Could you check a few things on this drawing? It's one solid part, dimensions in mm from its lowest x, y, z. A direction names the side the tool comes from. Round coordinates to 2 decimals unless told otherwise and drop trailing zeros. Order: outer loops, then holes, each group sorted by start corner. A loop starts at its lowest first (then second) coordinate and runs counter-clockwise, first axis right, second up.
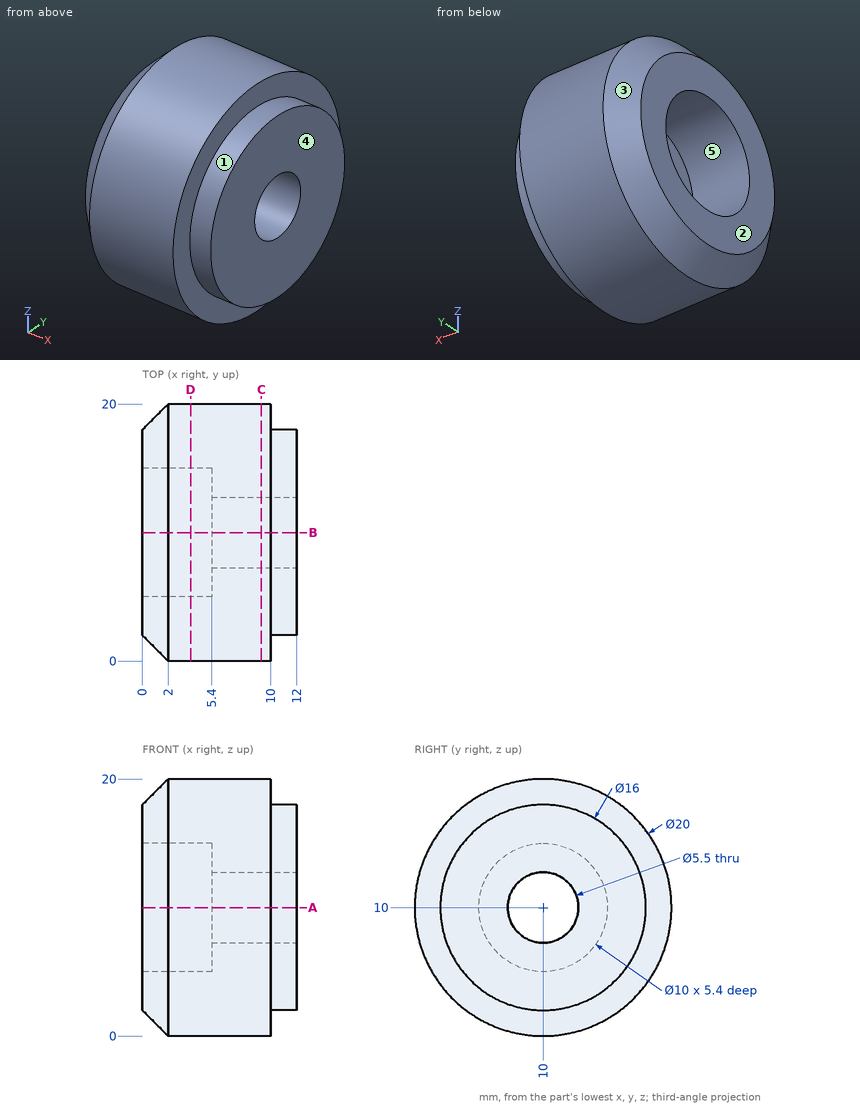
(1) On a 3-axis mill with a long thin cutter (end or side, diameter ignored), from which of +Z, -Z, +X, -X, +Y, -Y can I reach the whole of each face in a straight line? I mean the marked faces 1 and 2. Say none if no direction works.
(2) I'm going to push flat-ended pins straight in: pin 1 Ø3 at (x, y) = (3.5, 17.5) entering from -Z; pin 2 Ø2 at (y, z) = (16, 17) entering from +X; pin 3 Ø3 at (y, z) = (12, 8.5) entering from -X. Where does each tip first touch, or does it pass through?
(3) I want a section at C-C, the plane x = 9.25. List the corners of the cut face in (y, z) for me, plus the area to 3 significant figures.
(4) I want a section at D-D, the plane x = 3.75. List the corners of the cut face in (y, z) for me.
(5) Please list where these lines run through material, in increasing order: probe 1 along Y at (x, z) = (10.5, 10); probe 2 along Y at (x, z) = (7.5, 10); probe 3 along Z at (x, y) = (6.25, 7.75).
(6) If we mould it in two halves opening along Z, with no side actions, what happens to the marked faces 3, 4 and 5? For each: pulls with the +Z half, pulls with the -Z half, needs draft (parallel to the pull), parting line crosses it, or undercut.
(7) I want a section at A-A, the plane z = 10. List the corners of the cut face in (x, y) for me, plus the area to 3 significant figures.
Ans:
1. face 1: +X
1. face 2: +Z, -Z, -X, +Y, -Y
2. pin 1: stops at z = 2
2. pin 2: stops at x = 10
2. pin 3: stops at x = 5.4
3. outline: circle Ø20 at (10, 10); hole circle Ø5.5 at (10, 10)
3. area: 290 mm2
4. outline: circle Ø20 at (10, 10); hole circle Ø10 at (10, 10)
5. probe 1: y = 2 to 7.25, 12.75 to 18
5. probe 2: y = 0 to 7.25, 12.75 to 20
5. probe 3: z = 0.26 to 8.42, 11.58 to 19.74
6. face 3: parting line crosses it
6. face 4: needs draft
6. face 5: undercut
7. outline: (0, 2) - (2, 0) - (10, 0) - (10, 2) - (12, 2) - (12, 7.25) - (5.4, 7.25) - (5.4, 5) - (0, 5) - close; (0, 15) - (5.4, 15) - (5.4, 12.75) - (12, 12.75) - (12, 18) - (10, 18) - (10, 20) - (2, 20) - (0, 18) - close
7. area: 138 mm2
